Input: part model. Units: mm. Frame: model coordinates. Face numbers are marked on the shaded views. A direction names the side the tool comes from. Round coordinates to 2 decimals unless told otherwise and drop trailing zeros. Loops run counter-clockwise (first coordinate to the right, second up) from the corner with the lowest first, then second, coordinate; pieces in that order, holes last. Notation, with made-up numbers: M 12.25,85.5 L 54.25,85.5 A20 ccw 54.25,107.5 Z; hole C -18,-13.75 d1. An arc over 180 degrees is marked long. Use one line per item in the form item = value. Start each with the question number.
Q1. Ray query, line 1 along Z through (x, y) = (0, 2.7) (3 decimals); line 2 along X through (y, z) = (0.3, -9) (3 decimals); line 3 along Z through (x, y) = (8.5, 1.3) (3 decimals). Return the intervals inside material, ascending.
Q2. First-contact query: P1, Ø2.5, axis at x = 0, z = 23.05, coming from the -Y side; P2, Ø3, axis at x = 32.5, z = 32, coming from the +Y side (3 decimals); P3, Ø1.5, axis at x = -26, y = 4.5, coming from the +Z side. Flat tips, straight axial feed; report the tip coordinate or a pass-through.
Q3. Section query D-D, the plane x = -19. Output: boundary loops of the cut face in (y, z) (3 decimals), and give its area (3 significant figures).
Q4. Section query A-A, the plane x = 0. Output: boundary loops of the cut face in (y, z) (1 decimal), and give its area (3 significant figures).
Q5. Section query C-C, the plane y = 1.7. State how many separate pieces and enclosed holes the cut face has, and give its area (3 significant figures).
Q6. Access query for the marked faces 1 and 2. Directions: +Z, -Z, +X, -X, +Y, -Y. A direction counts if a zero-diameter tool reaches every point of the face in a straight line with its end or side. Return the directions, or none.
Q7. Section query B-B, the plane z = 0. Output: boundary loops of the cut face in (x, y) (1 decimal).
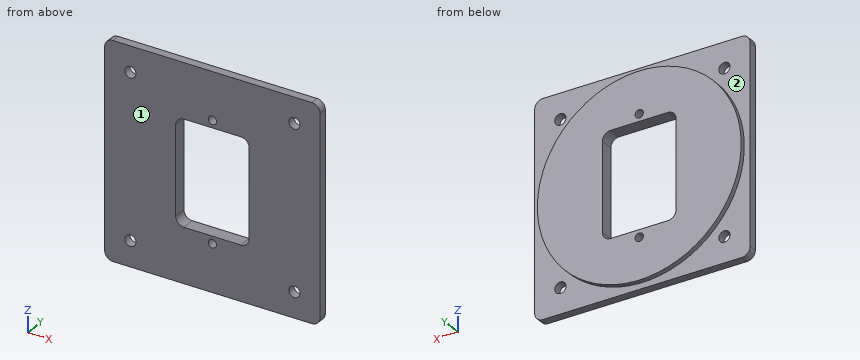
Autodesk Inventor part; units mm, degrees
ref_plane "YZ Plane" through (0, 0, 0) normal (1, 0, 0) x (0, 1, 0)
ref_plane "XZ Plane" through (0, 0, 0) normal (0, 1, 0) x (-1, 0, 0)
ref_plane "XY Plane" through (0, 0, 0) normal (0, 0, 1) x (1, 0, 0)
sketch "Sketch1" plane through (0, 0, 0) normal (0, 1, 0) x (-1, 0, 0)
  line L0 (41.275, 41.275) -> (-41.275, 41.275)
  line L1 (-41.275, 41.275) -> (-41.275, -41.275)
  line L2 (-41.275, -41.275) -> (41.275, -41.275)
  line L3 (41.275, -41.275) -> (41.275, 41.275)
  circle A0 centre (0, 0) radius 44.45 construction
  circle A1 centre (0, 0) radius 39.6875
  line L4 (-41.275, 41.275) -> (41.275, -41.275) construction
  line L5 (41.275, 41.275) -> (-41.275, -41.275) construction
  circle A2 centre (31.4309, 31.4309) radius 2.159
  circle A3 centre (31.4309, -31.4309) radius 2.159
  circle A4 centre (-31.4309, 31.4309) radius 2.159
  circle A5 centre (-31.4309, -31.4309) radius 2.159
  point P0 (0, 0)
  point P1 (0, 0)
  point P2 (0, 0)
  dimension "d0" = 82.55
  dimension "d1" = 82.55
  dimension "d2" = 88.9
  dimension "d3" = 79.375
  dimension "d4" = 4.318
  dimension "d5" = 4.318
  dimension "d6" = 4.318
  dimension "d7" = 4.318
extrude "Extrusion1" add sketch "Sketch1" along normal blind 3.175 contours L3 L2 L1 L0 | A1
sketch "Sketch2" plane through (0, 3.175, 0) normal (0, 1, 0) x (1, 0, 0)
  circle A0 centre (0, 0) radius 39.0525
  circle A1 centre (0, 0) radius 39.6875 construction
  line L0 (-14.097, -20.2057) -> (14.097, -20.2057)
  line L1 (14.097, -20.2057) -> (14.097, 20.2057)
  line L2 (14.097, 20.2057) -> (-14.097, 20.2057)
  line L3 (-14.097, 20.2057) -> (-14.097, -20.2057)
  line L4 (-14.097, -20.2057) -> (14.097, 20.2057) construction
  line L5 (14.097, -20.2057) -> (-14.097, 20.2057) construction
  circle A2 centre (0, -23.0505) radius 1.5875
  line L6 (-23.2122, 0) -> (23.719, 0) construction
  circle A3 centre (0, 23.0505) radius 1.5875
  point P0 (0, 0)
  dimension "d10" = 78.105
  dimension "d17" = 79.375
  dimension "d18" = 28.194
  dimension "d19" = 40.4114
  dimension "d21" = 3.175
  dimension "d24" = 46.101
extrude "Extrusion2" add sketch "Sketch2" along normal blind 1.905 contours A0 | L3 L2 L1 L0 | A2 | A3
fillet "Fillet1" radius 3.175 4 edges at (41.275, 1.5875, 41.275) (-41.275, 1.5875, 41.275) (-41.275, 1.5875, -41.275) (41.275, 1.5875, -41.275)
extrude "Extrusion3" cut sketch "Sketch2" along normal through all both and the other way through all contours L3 L2 L1 L0 | A2 | A3
fillet "Fillet5" radius 3.175 4 edges at (14.097, 2.54, 20.2057) (-14.097, 2.54, 20.2057) (-14.097, 2.54, -20.2057) (14.097, 2.54, -20.2057)
properties part number "ka51b-instrument-mount"
Results found:
q1.line_1 = -41.275 to -24.638, -21.463 to -20.206, 20.206 to 21.463, 24.638 to 41.275
q1.line_2 = -41.275 to -14.097, 14.097 to 41.275
q1.line_3 = -41.275 to -20.206, 20.206 to 41.275
q2.P1 = through
q2.P2 = 3.175
q2.P3 = 29.79
q3.outline = M 0,-41.275 L 3.175,-41.275 L 3.175,-34.119 L 5.08,-34.119 L 5.08,34.119 L 3.175,34.119 L 3.175,41.275 L 0,41.275 Z
q3.area = 392 mm²
q4.outline = M 0,-41.3 L 3.2,-41.3 L 3.2,-39.1 L 5.1,-39.1 L 5.1,-24.6 L 0,-24.6 Z; M 0,-21.5 L 5.1,-21.5 L 5.1,-20.2 L 0,-20.2 Z; M 0,20.2 L 5.1,20.2 L 5.1,21.5 L 0,21.5 Z; M 0,24.6 L 5.1,24.6 L 5.1,39.1 L 3.2,39.1 L 3.2,41.3 L 0,41.3 Z
q4.area = 173 mm²
q5.separate_pieces = 1
q5.enclosed_holes = 7
q5.area = 5,600 mm²
q6.face_1 = +Z, -Z, +X, -X, -Y
q6.face_2 = +Y
q7.outline = M -41.3,0 L -14.1,0 L -14.1,5.1 L -39.1,5.1 L -39.1,3.2 L -41.3,3.2 Z; M 14.1,0 L 41.3,0 L 41.3,3.2 L 39.1,3.2 L 39.1,5.1 L 14.1,5.1 Z
